For this review, use the dimensioned drawing (mm, ordinates from the lowest corner) and the shaded views. A direction names the side the tool comes from. Round coordinates to 2 decimals unless told otherwise and drop trailing zeros. Loops run counter-clockwise (first coordinate to the right, second up) from the corner with the lowest first, then second, coordinate; pieces in that order, holes last. Notation, with made-up numbers: (-38, 49) -> (14, 49) arc R21 cw to (14, 70) -> close; hole circle Ø3 at (-19.5, 52). An arc over 180 degrees is marked (long way). Answer as CSV lines item,"result". Start each with the question number.
(1) Take a section at D-D, the plane y = 11. Write out the cut boundary in (x, z), and give its area (3 significant figures).
(2) Take a section at B-B, the plane y = 7. Write out the cut boundary in (x, z), and give its area (3 significant figures).
(3) For P1, Ø6, axis at y = 11, z = 21, coming from the -X side; P2, Ø1.5, axis at x = 12.5, y = 10, coming from the -Z side; P3, Ø3, axis at x = 1.5, y = 11.5, coming from the +Z side, all flat-tipped, find the tip position at first contact; note any pin that passes through.
(4) Take a section at A-A, the plane x = 7. Write out the cut boundary in (y, z).
(5) Take a section at C-C, the plane z = 5.5. Write out the cut boundary in (x, y).
(6) To check wall thickness, follow line 1 (Z direction, x = 6.75, y = 6.5); line 2 (Z direction, x = 10.5, y = 10.75); line 3 (Y direction, x = 7.25, z = 25.5). State the ranges of each line that lie inside material, in increasing order. Write a range as from..to.
(7) Machinability: for the marked faces 1, 2 and 3, which of the approach directions +Z, -Z, +X, -X, +Y, -Y give a long, thin tool a straight path to every point of the face, cutting with its end or side? Answer none if there is none.
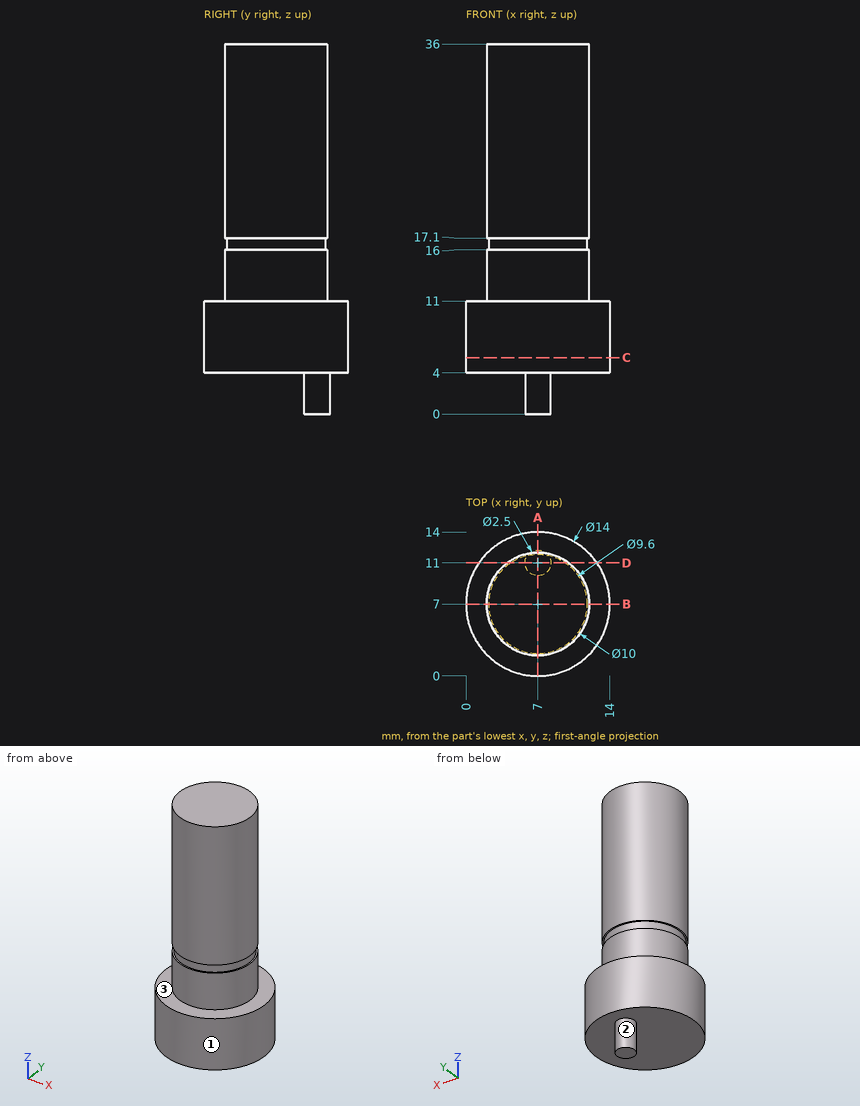
The answers:
1,outline,"(1.26, 4) -> (5.75, 4) -> (5.75, 0) -> (8.25, 0) -> (8.25, 4) -> (12.74, 4) -> (12.74, 11) -> (10, 11) -> (10, 16) -> (9.65, 16) -> (9.65, 17.1) -> (10, 17.1) -> (10, 36) -> (4, 36) -> (4, 17.1) -> (4.35, 17.1) -> (4.35, 16) -> (4, 16) -> (4, 11) -> (1.26, 11) -> close"
1,area,"240 mm²"
2,outline,"(0, 4) -> (14, 4) -> (14, 11) -> (12, 11) -> (12, 16) -> (11.8, 16) -> (11.8, 17.1) -> (12, 17.1) -> (12, 36) -> (2, 36) -> (2, 17.1) -> (2.2, 17.1) -> (2.2, 16) -> (2, 16) -> (2, 11) -> (0, 11) -> close"
2,area,"348 mm²"
3,P1,"x = 2.1"
3,P2,"z = 4"
3,P3,"z = 11"
4,outline,"(0, 4) -> (9.75, 4) -> (9.75, 0) -> (12.25, 0) -> (12.25, 4) -> (14, 4) -> (14, 11) -> (12, 11) -> (12, 16) -> (11.8, 16) -> (11.8, 17.1) -> (12, 17.1) -> (12, 36) -> (2, 36) -> (2, 17.1) -> (2.2, 17.1) -> (2.2, 16) -> (2, 16) -> (2, 11) -> (0, 11) -> close"
5,outline,"circle Ø14 at (7, 7)"
6,line 1,"4..36"
6,line 2,"4..11"
6,line 3,"2.01..11.99"
7,face 1,"+Z, -Z"
7,face 2,"-Z"
7,face 3,"+Z"
